```python
from build123d import *

# Parameters (mm, degrees)
SKETCH_1_R      = 1.75
SKETCH_1_W      = 22
SKETCH_1_H      = 42
EXTRUDE_1_DEPTH = 4
FILLET_1_R      = 5


with BuildPart() as part:
    # 草图1 → 凸台-拉伸1 (new body)
    with BuildSketch(Plane(origin=(0, 0, 0), x_dir=(1, 0, 0), z_dir=(0, 1, 0))):
        Polygon((-95, 52.5), (95, 52.5), (95, -28.5), (52, -28.5), (52, -52.5), (-95, -52.5), align=None)
        with Locations(Location((-89, -46.5, 0), (0, 0, 270))):
            Circle(SKETCH_1_R, mode=Mode.SUBTRACT)
        with Locations(Location((46, -46.5, 0), (0, 0, 270))):
            Circle(SKETCH_1_R, mode=Mode.SUBTRACT)
        with Locations(Location((46, 46.5, 0), (0, 0, 270))):
            Circle(SKETCH_1_R, mode=Mode.SUBTRACT)
        with Locations(Location((-89, 46.5, 0), (0, 0, 270))):
            Circle(SKETCH_1_R, mode=Mode.SUBTRACT)
        with Locations(Location((89, 46.5, 0), (0, 0, 270))):
            Circle(SKETCH_1_R, mode=Mode.SUBTRACT)
        with Locations(Location((89, -22.5, 0), (0, 0, 270))):
            Circle(SKETCH_1_R, mode=Mode.SUBTRACT)
        with Locations((68.5, 0)):
            Rectangle(SKETCH_1_W, SKETCH_1_H, mode=Mode.SUBTRACT)
    extrude(amount=EXTRUDE_1_DEPTH)

    # 圆角1
    fillet_1_edges = [part.edges().sort_by_distance(p)[0] for p in [
        (-95, 2, -52.5),
        (95, 2, -52.5),
        (95, 2, 28.5),
        (52, 2, 28.5),
        (52, 2, 52.5),
        (-95, 2, 52.5),
    ]]
    fillet(fillet_1_edges, radius=FILLET_1_R)


solid = part.part
```
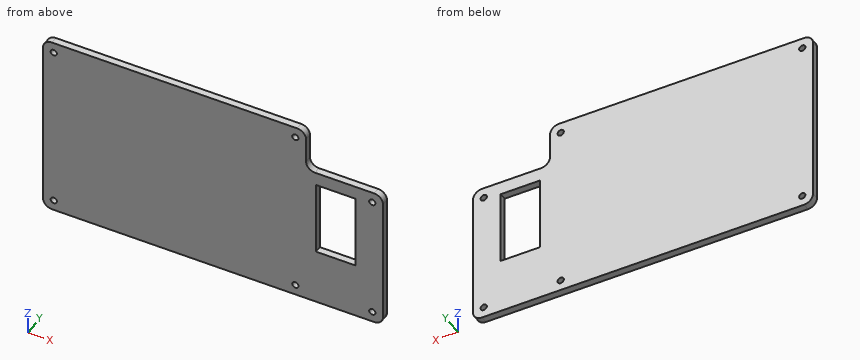
Read the model definition and answer for the solid it produces. Units are mm, in the model's axes. Coordinates: 2 decimals unless noted, no trailing zeros. Loops run counter-clockwise (first coordinate to the right, second up) from the corner with the lowest first, then second, coordinate; pieces in that order, holes last. Notation, with made-up numbers: (-10, 75.25) - (40, 75.25) arc R22 cw to (40, 87.25) - close; hole circle Ø5 at (24.5, 67). An arc over 180 degrees is marked (long way). Answer in a Markdown table with one row per item.
1. Find section A-A, the plane z = 10. Write down the section's boundary in (x, y).
Conclusion:
| item | result |
|---|---|
| outline | (-95, 0) - (57.5, 0) - (57.5, 4) - (-95, 4) - close; (79.5, 0) - (95, 0) - (95, 4) - (79.5, 4) - close |
2. Given pin 1 (2 mm diameter, centred on y = 1.5, z = 37.5, fed in from +X); pin 2 (2 mm diameter, centred on x = 66.5, y = 2.5, fed in from +Z), each flat-ended and moving along its own axis, determine where each tip first touches the part or whether it passes through.
Conclusion:
| item | result |
|---|---|
| pin 1 | stops at x = 52 |
| pin 2 | stops at z = 28.5 |
3. Find section B-B, the plane y = 1.5. Write down the section's boundary in (x, z).
Conclusion:
| item | result |
|---|---|
| outline | (-95, -47.5) arc R5 ccw to (-90, -52.5) - (90, -52.5) arc R5 ccw to (95, -47.5) - (95, 23.5) arc R5 ccw to (90, 28.5) - (57, 28.5) arc R5 cw to (52, 33.5) - (52, 47.5) arc R5 ccw to (47, 52.5) - (-90, 52.5) arc R5 ccw to (-95, 47.5) - close; hole circle Ø3.5 at (-89, -46.5); hole circle Ø3.5 at (-89, 46.5); hole circle Ø3.5 at (46, -46.5); hole circle Ø3.5 at (46, 46.5); hole (57.5, -21) - (79.5, -21) - (79.5, 21) - (57.5, 21) - close; hole circle Ø3.5 at (89, -46.5); hole circle Ø3.5 at (89, 22.5) |
4. Straight lines are drawn through the part: line 1 (X direction, y = 2.3, z = -46.5); line 2 (Z direction, x = 89, y = 2.45); line 3 (Z direction, x = -89, y = 2.5). For each, find the intervals that lie inside material, in ascending order.
Conclusion:
| item | result |
|---|---|
| line 1 | x = -95 to -90.75, -87.25 to 44.25, 47.75 to 87.25, 90.75 to 95 |
| line 2 | z = -52.5 to -48.25, -44.75 to 20.75, 24.25 to 28.5 |
| line 3 | z = -52.5 to -48.25, -44.75 to 44.75, 48.25 to 52.5 |
